from build123d import *

# Parameters (mm, degrees)
F0_W     = 60
F0_H     = 46
F1_DEPTH = 55
F1_TAPER = 5
F2_R     = 10


with BuildPart() as f1:
    # F0 (on Top) → F1 (new body)
    with BuildSketch(Plane.XY):
        Rectangle(F0_W, F0_H)
    extrude(amount=F1_DEPTH, taper=F1_TAPER)

    # F2
    f2_edges = [f1.edges().sort_by_distance(p)[0] for p in [
        (-27.594061, -20.594061, 27.500005),
        (27.594062, -20.594062, 27.5),
        (-27.594062, 20.594062, 27.5),
        (27.594061, 20.594061, 27.500005),
    ]]
    fillet(f2_edges, radius=F2_R)


solid = f1.part
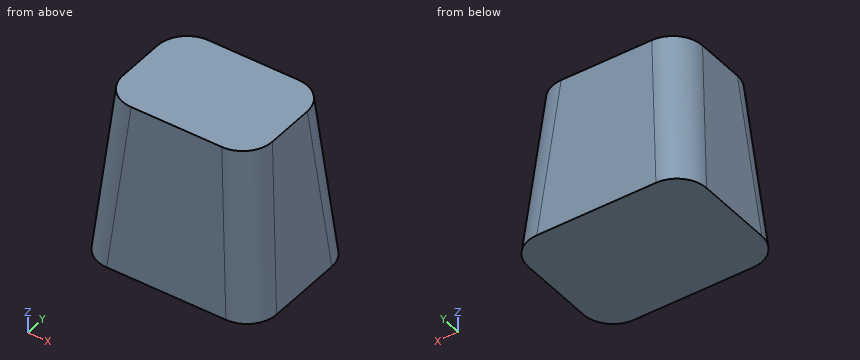
For this review, take the finished solid that the model builds, in its own axes (mm). Round coordinates to 2 decimals unless told otherwise and drop trailing zeros. Loops run counter-clockwise (first coordinate to the right, second up) from the corner with the lowest first, then second, coordinate; pieces in that order, holes last. Notation, with made-up numbers: (77.5, 86) - (87.5, 86) arc R7 ccw to (87.5, 97) - close; hole circle Ø10 at (10.25, 28.5). An arc over 180 degrees is marked (long way). Answer as CSV lines item,"result".
(1) Wall thickness on line 1 (X direction, y = 18.5, z = 16.5); line 2 (Y direction, x = -12, z = 14.5); line 3 (Y direction, x = -21, z = 6.5): over which ranges is each line inside the solid? List them lowest first.
Checked values:
line 1,"x = -25.78 to 25.78"
line 2,"y = -21.73 to 21.73"
line 3,"y = -22.31 to 22.31"
(2) Consider section B-B on y = 5. Give the boundary of the cut face in (x, z), then the cut area to 3 significant figures.
Checked values:
outline,"(-30, 0) - (30, 0) - (25.19, 55) - (-25.19, 55) - close"
area,"3,040 mm2"
(3) Insertion check: P1, Ø10, axis at y = -4.5, z = 13.5, coming from the +X side; P2, Ø8, axis at y = 4, z = 49, coming from the +X side; P3, Ø4, axis at x = 16.5, z = 26, coming from the +Y side. Each pin has a flat end and moves straight along its axis. Give the tip position at first contact, or say it passes through.
Checked values:
P1,"stops at x = 29.26"
P2,"stops at x = 26.06"
P3,"stops at y = 20.9"
(4) Consider section A-A on x = -1.5. Give the boundary of the cut face in (y, z), then the cut area to 3 significant figures.
Checked values:
outline,"(-23, 0) - (23, 0) - (18.19, 55) - (-18.19, 55) - close"
area,"2,270 mm2"
